Geometry check sheet. Reference: the model listing, model coordinates, mm. A direction names the side the tool comes from. Coordinates: 2 decimals unless noted, no trailing zeros. Write each loop counter-clockwise with the first axis right and the second up, starting at its lowest first coordinate (ties: lowest second). Pieces come first, ordered by that corner, then holes.
from build123d import *

# Parameters (mm, degrees)
SKETCH1_R           = 16.25
BOSS_EXTRUDE1_DEPTH = 35
SKETCH2_R           = 12.75
CUT_EXTRUDE1_DEPTH  = 35
SKETCH7_W           = 32.720020464
SKETCH7_H           = 16.591035764
CUT_EXTRUDE2_DEPTH  = 17.5
SKETCH9_W           = 32.5
SKETCH9_H           = 35
BOSS_EXTRUDE2_DEPTH = 7
SKETCH10_W          = 25.5
SKETCH10_H          = 35
CUT_EXTRUDE3_DEPTH  = 7
SKETCH15_R          = 2
CUT_EXTRUDE5_DEPTH  = 4
CUT_EXTRUDE6_START  = -4
SKETCH14_R          = 2
CUT_EXTRUDE6_DEPTH  = 4


with BuildPart() as part:
    # Sketch1 → Boss-Extrude1 (new body)
    with BuildSketch(Plane.XY):
        Circle(SKETCH1_R)
    extrude(amount=-BOSS_EXTRUDE1_DEPTH)

    # Sketch2 → Cut-Extrude1 (cut)
    with BuildSketch(Plane.XY):
        Circle(SKETCH2_R)
    extrude(amount=-CUT_EXTRUDE1_DEPTH, mode=Mode.SUBTRACT)

    # Sketch7 → Cut-Extrude2 (cut, symmetric)
    with BuildSketch(Plane.XY.offset(-17.5)):
        with Locations((-0.110010232, 8.295517882)):
            Rectangle(SKETCH7_W, SKETCH7_H)
    extrude(amount=CUT_EXTRUDE2_DEPTH, both=True, mode=Mode.SUBTRACT)

    # Sketch9 → Boss-Extrude2 (add)
    with BuildSketch(Plane(origin=(0, 0, 0), x_dir=(1, 0, 0), z_dir=(0, 1, 0))):
        with Locations((0, 17.5)):
            Rectangle(SKETCH9_W, SKETCH9_H)
    extrude(amount=BOSS_EXTRUDE2_DEPTH)

    # Sketch10 → Cut-Extrude3 (cut)
    with BuildSketch(Plane(origin=(0, 0, 0), x_dir=(1, 0, 0), z_dir=(0, 1, 0))):
        with Locations((0, 17.5)):
            Rectangle(SKETCH10_W, SKETCH10_H)
    extrude(amount=CUT_EXTRUDE3_DEPTH, mode=Mode.SUBTRACT)

    # Sketch15 → Cut-Extrude5 (cut)
    with BuildSketch(Plane(origin=(-16.25, 0, 0), x_dir=(0, 0, -1), z_dir=(1, 0, 0))):
        with Locations(Location((17.5, 0.25, 0), (0, 0, 187.180755781))):
            Circle(SKETCH15_R)
    extrude(amount=CUT_EXTRUDE5_DEPTH, mode=Mode.SUBTRACT)

    # Sketch14 → Cut-Extrude6 (cut)
    with BuildSketch(Plane(origin=(16.25, 0, 0), x_dir=(0, 0, -1), z_dir=(1, 0, 0)).offset(CUT_EXTRUDE6_START)):
        with Locations(Location((17.5, 0.25, 0), (0, 0, 187.180755781))):
            Circle(SKETCH14_R)
    extrude(amount=CUT_EXTRUDE6_DEPTH, mode=Mode.SUBTRACT)


solid = part.part
1. Sectioned sample at A-A, the plane z = -16. Record the boundary of the cut face in (x, y), and give its area (3 significant figures).
Computed values:
outline: (-16.25, 1.57) - (-12.75, 1.57) - (-12.75, 7) - (-16.25, 7) - close; (-16.21, -1.07) arc R16.25 ccw to (16.21, -1.07) - (12.7, -1.07) arc R12.75 cw to (-12.7, -1.07) - close; (12.75, 1.57) - (16.25, 1.57) - (16.25, 7) - (12.75, 7) - close
area: 190 mm2
2. Thickness scan on line 1 along X through (y, z) = (6, -24.5); line 2 along Z through (x, y) = (-15.25, 0.25). Record the ranges inside material, lowest first.
Computed values:
line 1: x = -16.25 to -12.75, 12.75 to 16.25
line 2: z = -35 to -19.5, -15.5 to 0
3. Sectioned sample at B-B, the plane y = -11.25. Record the boundary of the cut face in (x, z), and give its area (3 significant figures).
Computed values:
outline: (-11.73, -35) - (-6, -35) - (-6, 0) - (-11.73, 0) - close; (6, -35) - (11.73, -35) - (11.73, 0) - (6, 0) - close
area: 401 mm2
4. Access from +Z, -Z, +X, -X, +Y, -Y to the whole of each face (thin tool, end or side, straight path). Record for faces 4 (the flat face through (0, -13, 0)), 5 (the flat face through (-12.75, 3, -17)).
Computed values:
face 4: +Z, +X, -X, +Y, -Y
face 5: +Z, -Z, +Y
5. Sectioned sample at C-C, the plane z = -10.5. Record the boundary of the cut face in (x, y).
Computed values:
outline: (-16.25, 0) arc R16.25 ccw to (16.25, 0) - (16.25, 7) - (12.75, 7) - (12.75, 0) arc R12.75 cw to (-12.75, 0) - (-12.75, 7) - (-16.25, 7) - close
6. Draft check along X on faces 1 (the flat face through (16.25, 3, -17)), 2 (the cylindrical face through (-14.465, 0.413, -19.493)), 3 (the flat face through (12.75, 3, -17)). Enter one of: released by +X, released by -X, zero draft, split by the parting line, or undercut.
Computed values:
face 1: released by +X
face 2: zero draft
face 3: undercut
7. Gauge pin test, flat ends, axial feed: pin 1 Ø3 at (x, z) = (1, -10) entering from +Y; pin 2 Ø5 at (y, z) = (-8.5, -17.5) entering from -X; pin 3 Ø1 at (x, z) = (3.5, -24) entering from +Y. Record the tip position at first contact, or that the pin passes through.
Computed values:
pin 1: stops at y = -12.5
pin 2: stops at x = -15.1
pin 3: stops at y = -12.11
8. Sectioned sample at D-D, the plane y = 1.75. Record the boundary of the cut face in (x, z), and give its area (3 significant figures).
Computed values:
outline: (-16.25, -35) - (-12.75, -35) - (-12.75, -18.82) - (-16.25, -18.82) - close; (-16.25, -16.18) - (-12.75, -16.18) - (-12.75, 0) - (-16.25, 0) - close; (12.75, -35) - (16.25, -35) - (16.25, -18.82) - (12.75, -18.82) - close; (12.75, -16.18) - (16.25, -16.18) - (16.25, 0) - (12.75, 0) - close
area: 226 mm2
